For this review, take the finished solid that the model builds, in its own axes (mm). Face numbers are marked on the shaded views. A direction names the side the tool comes from. Give positions to 0.01 mm unless a question says otherwise; leave off trailing zeros. Loops run counter-clockwise (first coordinate to the right, second up) from the corner with the lowest first, then second, coordinate; pieces in that order, holes last. Notation, with made-up numbers: M -2,26 L 37,26 A6 ccw 37,34 Z; hole C -28.75,35.5 d7. An arc over 180 degrees is marked long. Use CSV: the item, a comma, the result in double quotes. Start each with the question number.
1. Take a section at D-D, the plane y = 10. Write out the cut boundary in (x, z).
2. The part is to be moulded in two halves that separate along Z. For the marked faces 1, 2, 3 and 4, say which applies: pulls with the +Z half, pulls with the -Z half, needs draft (parallel to the pull), parting line crosses it, or undercut.
3. Take a section at B-B, the plane x = 7.8. Write out the cut boundary in (y, z), and give its area (3 significant figures).
4. Take a section at A-A, the plane z = 15.4. Write out the cut boundary in (x, y).
5. Take a section at C-C, the plane z = 9.5. Write out the cut boundary in (x, y), and give its area (3 significant figures).
6. Insertion check: P1, Ø6, axis at x = 3, y = 9.5, coming from the -Z side; P2, Ø3.5, axis at y = 26, z = 12, coming from the -X side; P3, Ø2, axis at x = 16, y = 28, coming from the +Z side; P4, Ø2.5, axis at y = 23.9, z = 3.9, coming from the +X side. Each pin has a flat end and moves straight along its axis. Give the tip position at first contact, or say it passes through.
7. To check wall thickness, follow line 1 (Z direction, x = 16.9, y = 23.9); line 2 (Y direction, x = 14.5, z = 6.25); line 3 (Y direction, x = 5, z = 17). State the ranges of each line that lie inside material, in increasing order. Write a range as [from, to].
8. Tool access review of the marked faces 5, 6, 7, 8 and 9: name each direction out of +Z, -Z, +X, -X, +Y, -Y from which nothing blocks a thin tool from reaching the whole face with its end or side.
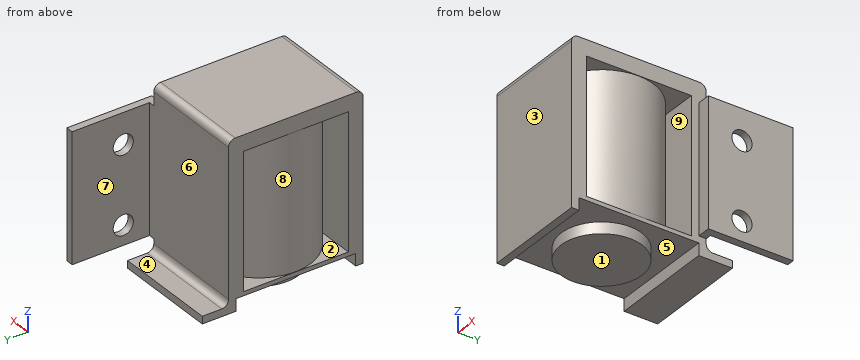
Solid Edge part; units mm, degrees
sketch "Sketch1" plane through (0, 0, 0) normal (0, 0, 1) x (1, 0, 0)
  line L0 (15.6, 20) -> (0, 20)
  line L1 (0, 20) -> (0, 0)
  line L2 (0, 0) -> (15.6, 0)
  line L3 (15.6, 0) -> (15.6, 20)
extrude "Protrusion1" add sketch "Sketch1" along normal blind 23
sketch "Sketch2" plane through (7.8, 10, 0) normal (0, 0, -1) x (0, 1, 0)
  circle A0 centre (0, 0) radius 6
extrude "ProtrusiónExtruida_2" add sketch "Sketch2" along normal blind 1.7
sketch "Sketch3" plane through (15.6, 10, 11.5) normal (1, 0, 0) x (0, 1, 0)
  line L0 (8.9, -13.3) -> (13.9, -13.3)
  line L1 (13.9, -13.3) -> (13.9, -12.2)
  line L2 (13.9, -12.2) -> (10, -12.2)
  line L3 (10, -12.2) -> (10, -11.5)
  line L4 (8.9, -11.5) -> (10, -11.5)
  line L5 (8.9, -11.5) -> (8.9, -13.3)
extrude "Protrusion2" add sketch "Sketch3" against normal up to surface (15.6 mm away)
sketch "Sketch4" plane through (15.6, 11.95, 10.6) normal (1, 0, 0) x (0, 1, 0)
  line L0 (6.95, -9.6) -> (6.95, 9.4)
  line L1 (6.95, 9.4) -> (8.05, 9.4)
  line L2 (8.05, 9.4) -> (8.05, -9.6)
  line L3 (8.05, -9.6) -> (6.95, -9.6)
extrude "ProtrusiónExtruida_4" add sketch "Sketch4" along normal blind 2
sketch "Sketch5" plane through (8.8, 20, 11.15) normal (0, 1, 0) x (-1, 0, 0)
  line L0 (-7.7, 8.85) -> (-7.7, -10.15)
  line L1 (-7.7, -10.15) -> (-8.8, -10.15)
  line L2 (-8.8, -10.15) -> (-8.8, 8.85)
  line L3 (-8.8, 8.85) -> (-7.7, 8.85)
extrude "ProtrusiónExtruida_5" add sketch "Sketch5" along normal blind 11.5
sketch "Sketch6" plane through (7.8, 9.45, 0) normal (0, 0, -1) x (0, 1, 0)
  line L0 (-8.35, -7.8) -> (-8.35, 7.8)
  line L1 (-8.35, 7.8) -> (-9.45, 7.8)
  line L2 (-9.45, 7.8) -> (-9.45, -7.8)
  line L3 (-9.45, -7.8) -> (-8.35, -7.8)
extrude "ProtrusiónExtruida_6" add sketch "Sketch6" along normal blind 1.8
sketch "Sketch7" plane through (17.6, 25.2, 10.5) normal (1, 0, 0) x (0, 1, 0)
  circle A0 centre (-1.3, 4.9) radius 1.5
  circle A1 centre (-1.3, -6.6) radius 1.5
extrude "Cutout1" cut sketch "Sketch7" against normal up to next
sketch "Sketch8" plane through (7.8, 10, 23) normal (0, 0, 1) x (1, 0, 0)
  line L0 (7.8, -7.8) -> (-7.8, -7.8)
  line L1 (-7.8, 7.8) -> (-7.8, -7.8)
  line L2 (7.8, 7.8) -> (-7.8, 7.8)
  line L3 (7.8, -7.8) -> (7.8, 7.8)
  circle A0 centre (0, 0) radius 7.75
extrude "Cutout2" cut sketch "Sketch8" against normal up to surface (20.05 mm away) from surface at -2.35
fillet "Redondeo_1" radius 1 3 edges at (7.8, 20, 23) (7.8, 0, 23) (7.8, 20, -0.7)
Result set:
1,outline,"M 0,0 L 1.8,0 L 1.8,-1.7 L 13.8,-1.7 L 13.8,0 L 15.6,0 L 15.6,0.6 L 15.55,0.6 L 15.55,20.65 L 15.6,20.65 L 15.6,23 L 0,23 L 0,20.65 L 0.05,20.65 L 0.05,0.6 L 0,0.6 Z"
2,face 1,"pulls with the -Z half"
2,face 2,"undercut"
2,face 3,"needs draft"
2,face 4,"pulls with the +Z half"
3,outline,"M 0,-1.8 L 1.1,-1.8 L 1.1,0 L 4,0 L 4,-1.7 L 16,-1.7 L 16,0 L 18.9,0 L 18.9,-1.8 L 23.9,-1.8 L 23.9,-0.7 L 21,-0.7 A1 cw 20,0.3 L 20,22 A1 ccw 19,23 L 1,23 A1 ccw 0,22 Z; hole M 2.2,0.6 L 2.25,0.6 L 2.25,20.65 L 2.2,20.65 Z; hole M 17.75,0.6 L 17.8,0.6 L 17.8,20.65 L 17.75,20.65 Z"
3,area,"486 mm2"
4,outline,"M 0,0 L 15.6,0 L 15.6,2.2 L 0,2.2 Z; M 0,17.8 L 15.6,17.8 L 15.6,18.9 L 17.6,18.9 L 17.6,22.4 L 16.5,22.4 L 16.5,20 L 0,20 Z; C 7.8,10 d15.5; M 16.5,25.4 L 17.6,25.4 L 17.6,31.5 L 16.5,31.5 Z"
5,outline,"M 0,0 L 15.6,0 L 15.6,2.2 L 0,2.2 Z; M 0,17.8 L 15.6,17.8 L 15.6,18.9 L 17.6,18.9 L 17.6,31.5 L 16.5,31.5 L 16.5,20 L 0,20 Z; C 7.8,10 d15.5"
5,area,"272 mm2"
6,P1,"z = -1.7"
6,P2,"x = 16.5"
6,P3,"z = 20"
6,P4,"through"
7,line 1,"[1, 2.4], [5.4, 13.9], [16.9, 20]"
7,line 2,"[0, 2.2], [6.1, 13.9], [17.8, 20]"
7,line 3,"[0, 2.2], [2.77, 17.23], [17.8, 20]"
8,face 5,"-Z"
8,face 6,"+Z, -X, +Y"
8,face 7,"+Z, -Z, -X, +Y"
8,face 8,"none"
8,face 9,"+X, -X"
